Here's how the part is built. I have some questions about the finished solid (model axes, mm). A direction names the side the tool comes from. Round coordinates to 2 decimals unless told otherwise and drop trailing zeros. Write each loop counter-clockwise with the first axis right and the second up, starting at its lowest first coordinate (ties: lowest second). Pieces come first, ordered by that corner, then holes. Notation, with made-up numbers: (-4.5, -15.75) - (37.5, -15.75) arc R28 cw to (37.5, 5.25) - close; hole circle Ø8 at (0, -15.75). An arc over 180 degrees is marked (long way). One line per item, written item: value. Start each with the question number.
Item 1: For P1, Ø3, axis at x = -1.5, y = -2.5, coming from the +Z side; P2, Ø1.3, axis at y = -1, z = -24, coming from the +X side; P3, Ø6, axis at x = -9.5, z = -5, coming from the -Y side; P4, Ø1.3, axis at x = -8, y = -2, coming from the +Z side, each with a flat end and sliding along its axis, tell me the tip position at first contact or that it passes through.
Item 2: Imagine slicing it at A-A, the plane z = -35.6. Please give me the cut outline in (x, y).
Item 3: Imagine slicing it at C-C, the plane y = 2.5. Please give me the cut outline in (x, z), then the cut area to 3 significant figures.
Item 4: For faces 5 (the face through (-6, 2, 0)), 6 (the face through (-9, -2, -10)), 7 (the face through (-6, -2, -20)), which set-ups out of +Z, -Z, +X, -X, +Y, -Y let a thin tool reach every point of the face, with its end or its side?
Item 5: Imagine slicing it at D-D, the plane x = -9.5. Please give me the cut outline in (y, z).
Item 6: If I drill on line 1 (Z direction, x = -3, y = 0.8); line 2 (X direction, y = 2.1, z = -35.6); line 3 (Z direction, x = -1.25, y = 1), over which ranges is the centre line in solid material (lowest first)?
Item 7: Thinking about a two-plate mould opening in Z: for faces 1 (the face through (-9, -4.4, -20)), 2 (the face through (-3.33, 2.03, -6.48)), 3 (the face through (-3.54, 2.03, -33.16)), 4 (the face through (-9, -2, -30)), which applies, released by +Z, released by -Z, zero draft, split by the parting line, or undercut?
Item 8: Imagine slicing it at B-B, the plane x = -3. Please give me the cut outline in (y, z).
Autodesk Inventor part; units mm, degrees
ref_plane "YZ Plane" through (0, 0, 0) normal (1, 0, 0) x (0, 1, 0)
ref_plane "XZ Plane" through (0, 0, 0) normal (0, 1, 0) x (-1, 0, 0)
ref_plane "XY Plane" through (0, 0, 0) normal (0, 0, 1) x (1, 0, 0)
sketch "Sketch1" plane through (0, 0, 0) normal (0, 1, 0) x (-1, 0, 0)
  line L0 (0, 0) -> (12, 0)
  line L1 (12, 0) -> (12, -40)
  line L2 (12, -40) -> (0, -40)
  line L3 (0, -40) -> (0, 0)
  dimension "d0" = 40
  dimension "d1" = 12
extrude "Extrusion1" add sketch "Sketch1" along normal blind 4
sketch "Sketch2" plane through (0, 4, 0) normal (0, 1, 0) x (1, 0, 0)
  circle A0 centre (-3, 4) radius 2.5
  circle A1 centre (-3, 35.6) radius 2.5
  line L0 (-12, 0) -> (0, 0)
  line L1 (0, 0) -> (0, 40)
  dimension "d4" = 5
  dimension "d5" = 5
  dimension "d6" = 4
  dimension "d7" = 3
  dimension "d8" = 31.6
  dimension "d9" = 3
extrude "Extrusion2" cut sketch "Sketch2" against normal blind 4
sketch "Sketch3" plane through (0, 0, 0) normal (0, -1, 0) x (1, 0, 0)
  line L0 (-12, -30) -> (-6, -30)
  line L1 (-6, -30) -> (-6, -10)
  line L2 (-6, -10) -> (-12, -10)
  line L3 (-12, -10) -> (-12, -30)
  line L4 (0, -40) -> (-12, -40)
  line L5 (-12, 0) -> (0, 0)
  line L6 (-12, -40) -> (-12, 0)
  dimension "d12" = 6
  dimension "d15" = 10
  dimension "d16" = 10
  dimension "d17" = 0
extrude "Extrusion3" add sketch "Sketch3" along normal blind 4.4
equation "\"d5\" = d4"
equation "\"d9\" = d7"
properties part number "B1 fermeture"
Values follow:
1. P1: passes through
1. P2: stops at x = -6
1. P3: stops at y = 0
1. P4: stops at z = -10
2. outline: (-12, 0) - (-5.5, 0) - (-5.5, 4) - (-12, 4) - close; (-0.5, 0) - (0, 0) - (0, 4) - (-0.5, 4) - close
3. outline: (-12, -40) - (0, -40) - (0, 0) - (-12, 0) - close; hole circle Ø5 at (-3, -35.6); hole circle Ø5 at (-3, -4)
3. area: 441 mm^2
4. face 5: +Z, +X, -X, +Y, -Y
4. face 6: +Z, +X, -X, -Y
4. face 7: +Z, -Z, +X, -Y
5. outline: (-4.4, -30) - (0, -30) - (0, -40) - (4, -40) - (4, 0) - (0, 0) - (0, -10) - (-4.4, -10) - close
6. line 1: z = -40 to -38.1, -33.1 to -6.5, -1.5 to 0
6. line 2: x = -12 to -5.5, -0.5 to 0
6. line 3: z = -40 to -37.39, -33.81 to -5.79, -2.21 to 0
7. face 1: zero draft
7. face 2: undercut
7. face 3: undercut
7. face 4: released by -Z
8. outline: (0, -40) - (4, -40) - (4, -38.1) - (0, -38.1) - close; (0, -33.1) - (4, -33.1) - (4, -6.5) - (0, -6.5) - close; (0, -1.5) - (4, -1.5) - (4, 0) - (0, 0) - close
